Work out the finished part from the listing and answer in its coordinate system (mm). A direction names the side the tool comes from. Coordinates: 2 decimals unless noted, no trailing zeros. Write each loop counter-clockwise with the first axis right and the second up, starting at its lowest first coordinate (ties: lowest second). Pieces come first, ordered by that corner, then holes. Notation, with made-up numbers: (10, -15.5) - (38, -15.5) arc R16 ccw to (38, -5.5) - close; hole circle Ø3 at (33, -28). An arc over 180 degrees is marked (long way). One line per item, written item: value.
```python
from build123d import *

# Parameters (mm, degrees)
SKETCH1_R           = 38.1
BOSS_EXTRUDE1_DEPTH = 12.7
SKETCH2_R           = 4.0005
CUT_EXTRUDE1_DEPTH  = 12.7
BOSS_EXTRUDE2_DEPTH = 12.7
SKETCH5_R           = 5.334
CUT_EXTRUDE2_DEPTH  = 2.54


with BuildPart() as part:
    # Sketch1 → Boss-Extrude1 (new body)
    with BuildSketch(Plane(origin=(0, 0, 0), x_dir=(1, 0, 0), z_dir=(0, 1, 0))):
        with Locations((-80.789858777, -8.415610289)):
            Circle(SKETCH1_R)
    extrude(amount=BOSS_EXTRUDE1_DEPTH)

    # Sketch2 → Cut-Extrude1 (cut)
    with BuildSketch(Plane(origin=(0, 12.7, 0), x_dir=(1, 0, 0), z_dir=(0, 1, 0))):
        with Locations((-80.789858777, -8.415610289)):
            Circle(SKETCH2_R)
    extrude(amount=-CUT_EXTRUDE1_DEPTH, mode=Mode.SUBTRACT)

    # Sketch3 → Boss-Extrude2 (add)
    with BuildSketch(Plane(origin=(0, 12.7, 0), x_dir=(1, 0, 0), z_dir=(0, 1, 0))):
        with BuildLine():
            ThreePointArc((-94.260242958, 5.054773892), (-88.079978163, 9.184294805), (-80.789858777, 10.634389711))
            Line((-80.789858777, 10.634389711), (-80.789858777, 29.684389711))
            ThreePointArc((-80.789858777, 29.684389711), (-95.37009755, 26.784199899), (-107.73062714, 18.525158074))
            Line((-107.73062714, 18.525158074), (-94.260242958, 5.054773892))
        make_face()
        with BuildLine():
            Line((-53.849090413, 18.525158074), (-67.319474595, 5.054773892))
            ThreePointArc((-67.319474595, 5.054773892), (-63.189953682, -1.125490903), (-61.739858777, -8.415610289))
            Line((-61.739858777, -8.415610289), (-42.689858777, -8.415610289))
            ThreePointArc((-42.689858777, -8.415610289), (-45.590048588, 6.164628484), (-53.849090413, 18.525158074))
        make_face()
        with BuildLine():
            Line((-53.849090413, -35.356378652), (-67.319474595, -21.885994471))
            ThreePointArc((-67.319474595, -21.885994471), (-73.49973939, -26.015515384), (-80.789858777, -27.465610289))
            Line((-80.789858777, -27.465610289), (-80.789858777, -46.515610289))
            ThreePointArc((-80.789858777, -46.515610289), (-66.209620003, -43.615420478), (-53.849090413, -35.356378652))
        make_face()
        with BuildLine():
            ThreePointArc((-94.260242958, -21.885994471), (-98.389763871, -15.705729676), (-99.839858777, -8.415610289))
            Line((-99.839858777, -8.415610289), (-118.889858777, -8.415610289))
            ThreePointArc((-118.889858777, -8.415610289), (-115.989668965, -22.995849062), (-107.73062714, -35.356378652))
            Line((-107.73062714, -35.356378652), (-94.260242958, -21.885994471))
        make_face()
    extrude(amount=BOSS_EXTRUDE2_DEPTH)

    # Sketch5 → Cut-Extrude2 (cut)
    with BuildSketch(Plane.XZ):
        with Locations((-80.789858777, 8.415610289)):
            Circle(SKETCH5_R)
    extrude(amount=-CUT_EXTRUDE2_DEPTH, mode=Mode.SUBTRACT)


solid = part.part
```
Item 1: Section C-C, the plane x = -111 is taken. Determine the outline of the cut face in (y, z), then the cut area to 3 significant figures.
Evaluation:
outline: (0, -14.8) - (12.7, -14.8) - (12.7, 8.42) - (25.4, 8.42) - (25.4, 31.63) - (0, 31.63) - close
area: 885 mm2
Item 2: Consider probe 1 along Z at (x, y) = (-81, 8); probe 2 along Y at (x, z) = (-47.5, 23); probe 3 along X at (y, z) = (15.75, 8). Determine where each line is inside the solid, lowest interval first.
Evaluation:
probe 1: z = -29.68 to 4.42, 12.41 to 46.52
probe 2: y = 0 to 12.7
probe 3: x = -61.74 to -42.69
Item 3: Section B-B, the plane z = 6 is taken. Determine the outline of the cut face in (x, y), then the cut area to 3 significant figures.
Evaluation:
outline: (-118.81, 0) - (-85.55, 0) - (-85.55, 2.54) - (-83.98, 2.54) - (-83.98, 12.7) - (-118.81, 12.7) - close; (-77.6, 2.54) - (-76.03, 2.54) - (-76.03, 0) - (-42.77, 0) - (-42.77, 25.4) - (-61.89, 25.4) - (-61.89, 12.7) - (-77.6, 12.7) - close
area: 1,120 mm2
Item 4: Determine the mould class of faces 5 (the face through (-107, 25.4, 19)), 6 (the face through (-101.09, 18.961, -11.884)), 7 (the face through (-77.094, 7.691, 9.948)) for opening direction X: +X half, -X half, draft (parallel to the pull), parting line (faces both ways), or undercut.
Evaluation:
face 5: draft
face 6: -X half
face 7: undercut
Item 5: Given pin 1 (14 mm diameter, centred on y = 17.5, z = 37, fed in from -X); pin 2 (6 mm diameter, centred on y = 15, z = -9, fed in from -X); pin 3 (8.5 mm diameter, centred on x = -80.5, z = 6.5, fed in from -Y); pin 4 (14 mm diameter, centred on x = -108, y = 19, fed in from -Z), each flat-ended and moving along its own axis, determine where each tip first touches the part or whether it passes through.
Evaluation:
pin 1: stops at x = -112.19
pin 2: stops at x = -115.6
pin 3: stops at y = 0
pin 4: stops at z = -23.88
Item 6: Section A-A, the plane y = 18.75 is taken. Determine the outline of the cut face in (x, z).
Evaluation:
outline: (-118.89, 8.42) - (-99.84, 8.42) arc R19.05 cw to (-94.26, 21.89) - (-107.73, 35.36) arc R38.1 ccw to start; (-107.73, -18.53) arc R38.1 ccw to (-80.79, -29.68) - (-80.79, -10.63) arc R19.05 cw to (-94.26, -5.05) - close; (-80.79, 27.47) arc R19.05 cw to (-67.32, 21.89) - (-53.85, 35.36) arc R38.1 ccw to (-80.79, 46.52) - close; (-67.32, -5.05) - (-53.85, -18.53) arc R38.1 ccw to (-42.69, 8.42) - (-61.74, 8.42) arc R19.05 cw to start
Item 7: Section D-D, the plane y = 4.75 is taken. Determine the outline of the cut face in (x, z), then the cut area to 3 significant figures.
Evaluation:
outline: circle Ø76.2 at (-80.79, 8.42); hole circle Ø8 at (-80.79, 8.42)
area: 4,510 mm2
Item 8: Which of the six approach directions +Z, -Z, +X, -X, +Y, -Y give full straight-line access (tool end or side, diameter ignored) to faces 1 (the face through (-80.79, 19, 37)), 2 (the face through (-109, 19, 8.416)), 3 (the face through (-52, 19, 8.416)), 4 (the face through (-80.79, 19, -20))?
Evaluation:
face 1: +Z, +Y
face 2: -X, +Y
face 3: +X, +Y
face 4: -Z, +Y
